The listing builds one solid part. Answer for the finished solid, in the listing's coordinates (mm). A direction names the side the tool comes from. Coordinates: 2 decimals unless noted, no trailing zeros. Loops run counter-clockwise (first coordinate to the right, second up) from the corner with the lowest first, then second, coordinate; pieces in that order, holes last. Notation, with made-up numbers: (8, -0.5) - (56, -0.5) arc R21 cw to (56, 22.5) - close; hole circle Ø1 at (65.25, 5). An arc over 180 degrees is marked (long way). Put each result on its own line as item: value.
Autodesk Inventor part; units mm, degrees
ref_plane "YZ Plane" through (0, 0, 0) normal (1, 0, 0) x (0, 1, 0)
ref_plane "XZ Plane" through (0, 0, 0) normal (0, 1, 0) x (-1, 0, 0)
ref_plane "XY Plane" through (0, 0, 0) normal (0, 0, 1) x (1, 0, 0)
sketch "Sketch1" plane through (0, 0, 0) normal (0, 1, 0) x (-1, 0, 0)
  line L0 (0, -21.336) -> (0, 21.336)
  line L1 (-21.336, 0) -> (21.336, 0)
  line L2 (15.24, -15.24) -> (4.191, -15.24)
  line L3 (-15.24, -15.24) -> (-4.191, -15.24)
  line L4 (15.24, 4.191) -> (12.827, 4.191)
  line L5 (12.827, -4.191) -> (15.24, -4.191)
  line L6 (-4.191, 12.827) -> (-4.191, 15.24)
  line L7 (4.191, 15.24) -> (4.191, 12.827)
  line L8 (-11.1208, -12.827) -> (-4.212, -5.9182)
  line L9 (-12.827, -11.1208) -> (-5.9182, -4.212)
  line L10 (-5.9182, 4.212) -> (-12.827, 11.1208)
  line L11 (-4.212, 5.9182) -> (-11.1208, 12.827)
  line L12 (-1.7062, 0) -> (0, 1.7062)
  line L13 (4.212, 5.9182) -> (11.1208, 12.827)
  line L14 (0, -1.7062) -> (1.7062, 0)
  line L15 (5.9182, 4.212) -> (12.827, 11.1208)
  line L16 (12.827, -11.1208) -> (5.9182, -4.212)
  line L17 (1.7062, 0) -> (0, 1.7062)
  line L18 (11.1208, -12.827) -> (4.212, -5.9182)
  line L19 (0, -1.7062) -> (-1.7062, 0)
  line L20 (4.191, -12.827) -> (4.191, -15.24)
  line L21 (-15.24, 4.191) -> (-12.827, 4.191)
  line L22 (-4.191, -15.24) -> (-4.191, -12.827)
  line L23 (-12.827, -4.191) -> (-15.24, -4.191)
  line L24 (11.1208, 12.827) -> (4.191, 12.827)
  line L25 (-4.191, 12.827) -> (-11.1208, 12.827)
  line L26 (-12.827, 11.1208) -> (-12.827, 4.191)
  line L27 (-12.827, -4.191) -> (-12.827, -11.1208)
  line L28 (-11.1208, -12.827) -> (-4.191, -12.827)
  line L29 (4.191, -12.827) -> (11.1208, -12.827)
  line L30 (12.827, -11.1208) -> (12.827, -4.191)
  line L31 (12.827, 4.191) -> (12.827, 11.1208)
  line L32 (-15.24, -15.24) -> (-15.24, -4.191)
  line L33 (-15.24, 4.191) -> (-15.24, 15.24)
  line L34 (15.24, -15.24) -> (4.191, -15.24)
  line L35 (-4.191, -15.24) -> (-15.24, -15.24)
  line L36 (15.24, 15.24) -> (15.24, 4.191)
  line L37 (15.24, -4.191) -> (15.24, -15.24)
  line L38 (-15.24, 15.24) -> (-4.191, 15.24)
  line L39 (4.191, 15.24) -> (15.24, 15.24)
  line L40 (4.212, 5.9182) -> (-4.212, 5.9182)
  line L41 (-5.9182, 4.212) -> (-5.9182, -4.212)
  line L42 (-4.212, -5.9182) -> (4.212, -5.9182)
  line L43 (5.9182, -4.212) -> (5.9182, 4.212)
  line L44 (5.9182, 5.9182) -> (-5.9182, -5.9182) construction
  line L45 (-5.9182, 5.9182) -> (5.9182, -5.9182) construction
  point P0 (0, 0)
  point P1 (0, -4.191)
  point P2 (-4.191, 0)
  point P3 (0, 4.191)
  point P4 (4.191, 0)
  dimension "d4" = 11.049
  dimension "d5" = 30.48
  dimension "d6" = 30.48
  dimension "d15" = 11.8364
  dimension "d16" = 11.8364
extrude "Extrusion1" add sketch "Sketch1" along normal blind 203.2 contours L42 L8 L28 L22 L3 L32 L23 L27 L9 L41 L1 L19 L0 | L0 L14 L1 L43 L16 L30 L5 L37 L2 L20 L29 L18 L42 | L17 L0 L40 L13 L24 L7 L39 L36 L4 L31 L15 L43 L1 | L1 L41 L10 L26 L21 L33 L38 L6 L25 L11 L40 L0 L12
properties part number "ProfileOne-01"
1) For faces 4 (the face through (-10, 100, -15.24)), 5 (the face through (-5.918, 100, 0)), determine the directions among +Z, -Z, +X, -X, +Y, -Y from which every point of the face is accessible in a straight line to the end or side of a thin tool.
Found:
face 4: -Z, +X, -X, +Y, -Y
face 5: -X, +Y, -Y
2) For a pull along X with two mould halves and no side action, classify faces 1 (the face through (10, 100, 15.24)), 2 (the face through (12.827, 100, -8)), 3 (the face through (5.918, 100, 0)) as pulls with the +X half, pulls with the -X half, needs draft (parallel to the pull), parting line crosses it, or undercut.
Found:
face 1: needs draft
face 2: undercut
face 3: pulls with the +X half
3) Each of these flat-tipped pins is pushed along its axis until it touches: pin 1 (4 mm diameter, centred on x = 2.5, z = 8, fed in from -Y); pin 2 (6.5 mm diameter, centred on y = 137, z = 0.5, fed in from -X). Where does it stop, or does it pass through?
Found:
pin 1: passes through
pin 2: stops at x = -5.92
4) The part is cut by section A-A (z = -8). Give the vertices of the cut face in (x, y).
Found:
outline: (-15.24, 0) - (-12.83, 0) - (-12.83, 203.2) - (-15.24, 203.2) - close; (-9.71, 0) - (-6.29, 0) - (-6.29, 203.2) - (-9.71, 203.2) - close; (6.29, 0) - (9.71, 0) - (9.71, 203.2) - (6.29, 203.2) - close; (12.83, 0) - (15.24, 0) - (15.24, 203.2) - (12.83, 203.2) - close
5) The part is cut by section B-B (x = -8). Give the vertices of the cut face in (y, z), and give its area (3 significant figures).
Found:
outline: (0, -15.24) - (203.2, -15.24) - (203.2, -12.83) - (0, -12.83) - close; (0, -9.71) - (203.2, -9.71) - (203.2, -6.29) - (0, -6.29) - close; (0, 6.29) - (203.2, 6.29) - (203.2, 9.71) - (0, 9.71) - close; (0, 12.83) - (203.2, 12.83) - (203.2, 15.24) - (0, 15.24) - close
area: 2,370 mm^2
6) Straight lines are drawn through the part: L1, parallel to X at y = 145.5, z = 0; L2, parallel to Z at x = 7.5, y = 94; L3, parallel to X at y = 113, z = -5. For each, find the intervals that lie inside material, in ascending order. Write a range as [from, to].
Found:
L1: x = [-5.92, -1.71], [1.71, 5.92]
L2: z = [-15.24, -12.83], [-9.21, -5.79], [5.79, 9.21], [12.83, 15.24]
L3: x = [-15.24, -12.83], [-6.71, 6.71], [12.83, 15.24]
